Check sheet for the modelled part. Datum: model origin and axes. Units: mm. A direction names the side the tool comes from. Give positions to 0.01 mm unless a question says otherwise; leave off trailing zeros. Write each loop counter-clockwise with the first axis right and the second up, starting at its lowest first coordinate (ties: lowest second). Pieces come first, ordered by that corner, then holes. Notation, with made-up numbers: (86.5, -37.75) -> (114.5, -37.75) arc R13 ccw to (114.5, -27.75) -> close; hole circle Ø10 at (85, 35.5). An arc over 180 degrees is marked (long way). Use a Markdown table: item, result. Add a question column.
1. Set-up check for faces 4 (the flat face through (-14, -13, 19.626)), 5 (the flat face through (-74.408, -15.344, 26.754)): record each of +Z, -Z, +X, -X, +Y, -Y from which the full face is reachable in a straight line by a thin tool's end or side.
2. Scan lines: probe 1 along Z at (x, y) = (-25, -20); probe 2 along X at (y, z) = (-15.25, 32.25); probe 3 along X at (y, z) = (-23.5, 20.75). Record each from-to range of solid material in increasing order. Write a range as [from, to].
3. Cross-section at B-B (z = 34). Enter the section's corners in (x, y), then the cut area to 3 significant figures.
4. Cross-section at A-A (y = -5.25). Enter the section's corners in (x, z).
5. Gauge pin test, flat ends, axial feed: P1, Ø1.5, axis at x = -14, z = 20, coming from the -Y side; P2, Ø1.5, axis at y = -5.5, z = 27, coming from the -X side; P3, Ø12, axis at y = -5, z = 32.5, coming from the +X side. Record the tip position at first contact, or that the pin passes through.
6. Cross-section at C-C (x = -59). Enter the section's corners in (y, z), then the cut area to 3 significant figures.
7. Release check for a two-part mould opening along Z. For faces 1 (the flat face through (-16, -13, 16.451)), 2 (the flat face through (-8, 0, 19)), 3 (the cylindrical face through (-74.58, -12.42, 29.07)) record: released by +Z, released by -Z, zero draft, split by the parting line, or undercut.
from build123d import *

# Parameters (mm, degrees)
F1_DEPTH = 25.4
F2_R     = 2.15265
F4_DEPTH = 25.4
F3_R     = 2.15265
F5_DEPTH = 25.4


with BuildPart() as f1:
    # F0 (on Front) → F1 (new body)
    with BuildSketch(Plane.XZ):
        Polygon((-66.6809173423, 16.451433301), (35.5159826577, 16.451433301), (65.9959826577, 39.311433301), (64.4719826577, 41.343433301), (35.5159826577, 19.626433301), (-65.8871673423, 19.626433301), (-79.8889173423, 38.295433301), (-81.9209173423, 36.771433301), align=None)
    extrude(amount=F1_DEPTH)

    # F2 (on face) → F4 (cut)
    with BuildSketch(Plane(origin=(4.8890657723, 0, -6.5187543631), x_dir=(0.8, 0, 0.6), z_dir=(0.6, 0, -0.8))):
        with Locations((58.1185061067, 12.7)):
            Circle(F2_R)
    extrude(amount=-F4_DEPTH, mode=Mode.SUBTRACT)

    # F3 (on face) → F5 (cut)
    with BuildSketch(Plane(origin=(-34.7790991146, 0, -26.084324336), x_dir=(0, -1, 0), z_dir=(-0.8, 0, -0.6))):
        with Locations((12.7, 65.8696970462)):
            Circle(F3_R)
    extrude(amount=-F5_DEPTH, mode=Mode.SUBTRACT)


solid = f1.part
Worked answers:
| question | item | result |
|---|---|---|
| 1 | face 4 | +Z, +Y, -Y |
| 1 | face 5 | -Z, -X, +Y, -Y |
| 2 | probe 1 | z = [16.45, 19.63] |
| 2 | probe 2 | x = [-78.53, -75.35], [52.35, 56.58] |
| 2 | probe 3 | x = [-69.9, -66.73], [37.01, 41.25] |
| 3 | outline | (-79.84, -25.4) -> (-76.67, -25.4) -> (-76.67, 0) -> (-79.84, 0) -> close; (54.68, -25.4) -> (58.91, -25.4) -> (58.91, 0) -> (54.68, 0) -> close |
| 3 | area | 188 mm² |
| 4 | outline | (-81.92, 36.77) -> (-66.68, 16.45) -> (35.52, 16.45) -> (66, 39.31) -> (64.47, 41.34) -> (35.52, 19.63) -> (-65.89, 19.63) -> (-79.89, 38.3) -> close |
| 5 | P1 | stops at y = -25.4 |
| 5 | P2 | stops at x = -75.15 |
| 5 | P3 | stops at x = 64.91 |
| 6 | outline | (-25.4, 16.45) -> (0, 16.45) -> (0, 19.63) -> (-25.4, 19.63) -> close |
| 6 | area | 80.6 mm² |
| 7 | face 1 | released by -Z |
| 7 | face 2 | zero draft |
| 7 | face 3 | undercut |
